Here's how the part is built. I have some questions about the finished solid (model axes, mm). A direction names the side the tool comes from. Give positions to 0.01 mm unless a question says otherwise; leave off trailing zeros. Write each loop counter-clockwise with the first axis right and the second up, starting at its lowest first coordinate (ties: lowest second). Pieces come first, ordered by that corner, then holes. Notation, with made-up numbers: (87, 1) - (141, 1) arc R16 cw to (141, 5) - close; hole circle Ø4 at (35, -5). An arc over 180 degrees is marked (long way). Write each question's results on one line, items separated by ' | '. Start each with the question number.
Item 1: Suppose I cut it at D-D on x = 63. List the corners of the cut face in (y, z) for me, then the cut area to 3 significant figures.
Item 2: Suppose I cut it at A-A on x = 23. List the corners of the cut face in (y, z) for me.
Item 3: Please list where these lines run through material, in increasing order: line 1 along Y through (x, z) = (43.5, -4.5); line 2 along X through (y, z) = (4, -2.5); line 3 along X through (y, z) = (-6, -6.5).
Item 4: Suppose I cut it at B-B on z = 4. Count the separate pieces of the cut face and the enclosed holes in it, then the cut area to 3 significant figures.
Item 5: We'd pull the mould along Z, two halves only. Please class faces 1 (the flat face through (69, 0, -8)), 2 (the flat face through (50, 0, -6)), 3 (the flat face through (69, 0, 8)), 4 (the flat face through (53.5, -2, 0.1)): +Z half, -Z half, draft (parallel to the pull), parting line (faces both ways), or undercut.
Item 6: Which directions (+Z, -Z, +X, -X, +Y, -Y) give clear straight access to the entire face, cutting with the end or side of a thin tool? Please do faces 5 (the flat face through (63, 2, 0)), 6 (the flat face through (59, 0, 0)), 7 (the flat face through (40, 0, -10)).
Item 7: Will these pins go through, and if not, where does the flat tip stop? P1, Ø1, axis at y = 8, z = -2, coming from the +X side; P2, Ø2, axis at y = 0.5, z = -2, coming from the -X side; P3, Ø4, axis at y = 2, z = 5, coming from the -X side.
Item 8: Suppose I cut it at C-C on y = 7.5. List the corners of the cut face in (x, z) for me.
```python
from build123d import *

# Parameters (mm, degrees)
F1_DEPTH = 10
F2_W     = 3
F2_H     = 12
F3_DEPTH = 10
F5_SIZE  = 3
F6_R     = 8


with BuildPart() as f1:
    # F0 (on Top) → F1 (new body, symmetric)
    with BuildSketch(Plane.XY):
        with BuildLine():
            ThreePointArc((43.370497, 2), (37.315196, 4.041776), (33.732609, 9.333333))
            ThreePointArc((33.732609, 9.333333), (30.149158, 17.777184), (24.494897, 25))
            Line((24.494897, 25), (19.974984, 25))
            ThreePointArc((19.974984, 25), (32, 0), (19.974984, -25))
            Line((19.974984, -25), (24.494897, -25))
            ThreePointArc((24.494897, -25), (30.149158, -17.777184), (33.732609, -9.333333))
            ThreePointArc((33.732609, -9.333333), (37.315196, -4.041776), (43.370497, -2))
            Line((43.370497, -2), (70, -2))
            Line((70, -2), (70, 2))
            Line((70, 2), (43.370497, 2))
        make_face()
    extrude(amount=F1_DEPTH, both=True)


with BuildPart() as f3:
    # F2 (on Front) → F3 (new body, symmetric)
    with BuildSketch(Plane.XZ):
        with Locations((65.5, 0)):
            Rectangle(F2_W, F2_H)
        with Locations((45.5, 0)):
            Rectangle(F2_W, F2_H)
        with Locations((50.5, 0)):
            Rectangle(F2_W, F2_H)
        with Locations((60.5, 0)):
            Rectangle(F2_W, F2_H)
        with Locations((55.5, 0)):
            Rectangle(F2_W, F2_H)
        with Locations((35.5, 0)):
            Rectangle(F2_W, F2_H)
    extrude(amount=F3_DEPTH, both=True)


with BuildPart() as f1_1:
    add(f1.part)

    # F4: cut F3
    add(f3.part, mode=Mode.SUBTRACT)

    # F5
    f5_edges = [f1_1.edges().sort_by_distance(p)[0] for p in [
        (70, 0, 10),
        (70, 0, -10),
    ]]
    chamfer(f5_edges, length=F5_SIZE)

    # F6
    f6_edges = [f1_1.edges().sort_by_distance(p)[0] for p in [
        (24.494897, 25, 0),
        (24.494897, -25, 0),
    ]]
    fillet(f6_edges, radius=F6_R)


solid = f1_1.part
```
Checked values:
1) outline: (-2, -10) - (2, -10) - (2, 10) - (-2, 10) - close | area: 80.0 mm^2
2) outline: (-24.74, -10) - (-22.25, -10) - (-22.25, 10) - (-24.74, 10) - close; (22.25, -10) - (24.74, -10) - (24.74, 10) - (22.25, 10) - close
3) line 1: y = -2 to 2 | line 2: x = 31.75 to 34, 37 to 37.37 | line 3: x = 31.43 to 35.37
4) separate pieces: 7 | enclosed holes: 0 | area: 236 mm^2
5) face 1: -Z half | face 2: undercut | face 3: +Z half | face 4: draft
6) face 5: +Z, -Z, +X, +Y | face 6: +Y, -Y | face 7: -Z, +X, -X, +Y, -Y
7) P1: stops at x = 34 | P2: stops at x = 31.96 | P3: stops at x = 31.75
8) outline: (31.11, -10) - (34.44, -10) - (34.44, -6) - (34, -6) - (34, 6) - (34.44, 6) - (34.44, 10) - (31.11, 10) - close
